Geometry: final body of the model. Coordinates: model frame, mm. A direction names the side the tool comes from. Round coordinates to 2 decimals unless told otherwise and drop trailing zeros. Loops run counter-clockwise (first coordinate to the right, second up) from the corner with the lowest first, then second, coordinate; pieces in that order, holes last. Notation, with made-up numbers: (-23, -36.75) - (32, -36.75) arc R17 ccw to (32, -24.75) - close; hole circle Ø1 at (27.5, 62). An arc over 180 degrees is marked (long way). Use CSV: the item, a comma, the result in double quotes.
from build123d import *

# Parameters (mm, degrees)
SKETCH1_W               = 50.8
SKETCH1_H               = 76.2
BASE_FLANGE1_DEPTH      = 3.175
EDGE_FLANGE1_DEPTH      = 76.2
F_1_4_CLEARANCE_HOLE1_D = 6.7564
F_1_4_CLEARANCE_HOLE2_D = 6.7564


# Sheet-metal steps are written as plain solids
with BuildPart() as part:
    # Sketch1 → Base-Flange1 (new body)
    with BuildSketch(Plane.XY):
        with Locations((25.4, 38.1)):
            Rectangle(SKETCH1_W, SKETCH1_H)
    extrude(amount=-BASE_FLANGE1_DEPTH)

    # Edge-Flange1 section (across the edge) → Edge-Flange1 (add)
    with BuildSketch(Plane(origin=(52.324, 0, 0), x_dir=(-1, 0, 0), z_dir=(0, 1, 0))):
        with BuildLine():
            Line((-3.175, 1.524), (-3.175, 50.8))
            Line((-3.175, 50.8), (0, 50.8))
            Line((0, 50.8), (0, 1.524))
            ThreePointArc((0, 1.524), (0.446369265, 0.446369265), (1.524, 0))
            Line((1.524, 0), (1.524, -3.175))
            ThreePointArc((1.524, -3.175), (-1.798694765, -1.798694765), (-3.175, 1.524))
        make_face()
    extrude(amount=EDGE_FLANGE1_DEPTH)

    # 1/4 Clearance Hole1 (through all)
    with Locations(Plane.XY):
        with Locations((38.1, 63.5), (12.7, 63.5), (12.7, 38.1), (38.1, 38.1), (12.7, 12.7), (38.1, 12.7)):
            Hole(F_1_4_CLEARANCE_HOLE1_D / 2)

    # 1/4 Clearance Hole2 (through all)
    with Locations(Plane.ZY.offset(-52.324)):
        with Locations((13.462, 63.5), (38.862, 63.5), (13.462, 38.1), (38.862, 38.1), (13.462, 12.7), (38.862, 12.7)):
            Hole(F_1_4_CLEARANCE_HOLE2_D / 2)


solid = part.part
Item 1: Section C-C on y = 53. Return the cut outline in (x, z) (3 decimals).
Final values:
outline,"(0, -3.175) - (50.8, -3.175) arc R4.699 ccw to (55.499, 1.524) - (55.499, 50.8) - (52.324, 50.8) - (52.324, 1.524) arc R1.524 cw to (50.8, 0) - (0, 0) - close"
Item 2: Section A-A on x = 12.7. Return the cut outline in (y, z) (3 decimals).
Final values:
outline,"(0, -3.175) - (9.322, -3.175) - (9.322, 0) - (0, 0) - close; (16.078, -3.175) - (34.722, -3.175) - (34.722, 0) - (16.078, 0) - close; (41.478, -3.175) - (60.122, -3.175) - (60.122, 0) - (41.478, 0) - close; (66.878, -3.175) - (76.2, -3.175) - (76.2, 0) - (66.878, 0) - close"
Item 3: Section D-D on z = 19.5. Return the cut outline in (x, y).
Final values:
outline,"(52.32, 0) - (55.5, 0) - (55.5, 76.2) - (52.32, 76.2) - close"
Item 4: Section B-B on y = 63.5. Return the cut outline in (x, z) (3 decimals), plus the area to 3 significant figures.
Final values:
outline,"(0, -3.175) - (9.322, -3.175) - (9.322, 0) - (0, 0) - close; (16.078, -3.175) - (34.722, -3.175) - (34.722, 0) - (16.078, 0) - close; (41.478, -3.175) - (50.8, -3.175) arc R4.699 ccw to (55.499, 1.524) - (55.499, 10.084) - (52.324, 10.084) - (52.324, 1.524) arc R1.524 cw to (50.8, 0) - (41.478, 0) - close; (52.324, 16.84) - (55.499, 16.84) - (55.499, 35.484) - (52.324, 35.484) - close; (52.324, 42.24) - (55.499, 42.24) - (55.499, 50.8) - (52.324, 50.8) - close"
area,"247 mm²"
Item 5: Material intervals for line 1 (Y direction, x = 12.7, z = -2.2); line 2 (Z direction, x = 33, y = 37) (3 decimals); line 3 (X direction, y = 11, z = 31.5), sorted ascending.
Final values:
line 1,"y = 0 to 9.32, 16.08 to 34.72, 41.48 to 60.12, 66.88 to 76.2"
line 2,"z = -3.175 to 0"
line 3,"x = 52.32 to 55.5"
Item 6: Reachability of faces 5 (the flat face through (25, 39, 0)), 6 (the cylindrical face through (13.43, 60.2, -1.61)) from +Z, -Z, +X, -X, +Y, -Y: full face, straight path, thin tool, end or side. Return the list, or none.
Final values:
face 5,"+Z, -X, +Y, -Y"
face 6,"+Z, -Z"
Item 7: Mould query, pull axis Y, two halves, no side actions, for faces 1 (the flat face through (36, 76.2, -2)), 2 (the cylindrical face through (41.475, 12.849, -1.61)), 3 (the flat face through (0, 38, -2)), 4 (the flat face through (36, 0, -2)). Classes: released by +Y, released by -Y, zero draft, split by the parting line, or undercut.
Final values:
face 1,"released by +Y"
face 2,"undercut"
face 3,"zero draft"
face 4,"released by -Y"
Item 8: Pin query (flat end, axial travel): P1, Ø8, axis at x = 38.1, y = 63.5, coming from the +Z side; P2, Ø6, axis at y = 12.7, z = 38.862, coming from the +X side; P3, Ø8, axis at y = 48, z = 9, coming from the -X side. Return the tip coordinate at first contact, or that it passes through.
Final values:
P1,"stops at z = 0"
P2,"passes through"
P3,"stops at x = 52.32"
